from build123d import *

# Parameters (mm, degrees)
SKETCH_1_R          = 10
SKETCH_1_R_2        = 3.5
SKETCH_1_R_3        = 1.5
EXTRUDE_1_DEPTH     = 3
SKETCH_2_R          = 10
SKETCH_2_R_2        = 4.5
SKETCH_2_R_3        = 1.5
CUT_EXTRUDE_1_DEPTH = 1


with BuildPart() as part:
    # 草图1 → 凸台-拉伸1 (new body)
    with BuildSketch(Plane(origin=(0, 0, 0), x_dir=(1, 0, 0), z_dir=(0, 1, 0))):
        Circle(SKETCH_1_R)
        Circle(SKETCH_1_R_2, mode=Mode.SUBTRACT)
        with Locations((0, 6.5)):
            Circle(SKETCH_1_R_3, mode=Mode.SUBTRACT)
        with Locations((0, -6.5)):
            Circle(SKETCH_1_R_3, mode=Mode.SUBTRACT)
        with Locations((-6.5, 0)):
            Circle(SKETCH_1_R_3, mode=Mode.SUBTRACT)
        with Locations((6.5, 0)):
            Circle(SKETCH_1_R_3, mode=Mode.SUBTRACT)
    extrude(amount=EXTRUDE_1_DEPTH)

    # 草图2 → 切除-拉伸1 (cut)
    with BuildSketch(Plane(origin=(0, 3, 0), x_dir=(1, 0, 0), z_dir=(0, 1, 0))):
        Circle(SKETCH_2_R)
        Circle(SKETCH_2_R_2, mode=Mode.SUBTRACT)
        with Locations((0, -6.5)):
            Circle(SKETCH_2_R_3, mode=Mode.SUBTRACT)
        with Locations((0, 6.5)):
            Circle(SKETCH_2_R_3, mode=Mode.SUBTRACT)
        with Locations((6.5, 0)):
            Circle(SKETCH_2_R_3, mode=Mode.SUBTRACT)
        with Locations((-6.5, 0)):
            Circle(SKETCH_2_R_3, mode=Mode.SUBTRACT)
    extrude(amount=-CUT_EXTRUDE_1_DEPTH, mode=Mode.SUBTRACT)


solid = part.part
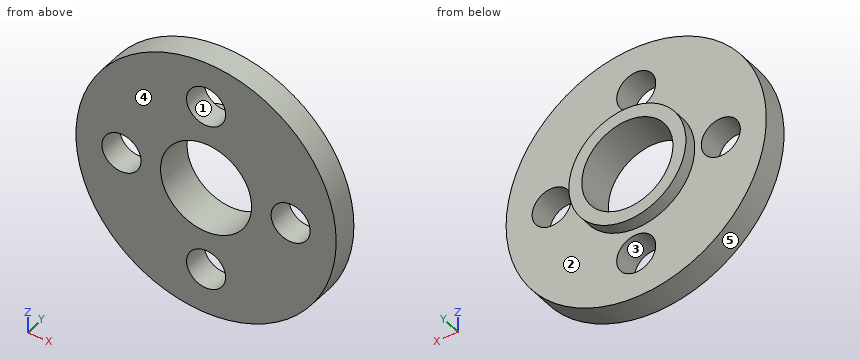
Design review of the part built by this model. Coordinates are the model's own, in mm. Face numbers are marked on the shaded views. A direction names the side the tool comes from. Coordinates: 2 decimals unless noted, no trailing zeros. Loops run counter-clockwise (first coordinate to the right, second up) from the corner with the lowest first, then second, coordinate; pieces in that order, holes last. Notation, with made-up numbers: (43, -36) -> (65, -36) arc R21 cw to (65, -29) -> close; hole circle Ø3 at (-29, -36). An arc over 180 degrees is marked (long way). Use a Markdown table: item, result. Add a question column.
Item 1: Clearance check with flat-ended pins moving along their axes: P1, Ø1.5, axis at x = 0.5, z = 6.5, coming from the +Y side; P2, Ø4, axis at x = 3, z = 7.5, coming from the +Y side; P3, Ø1, axis at y = 0.5, z = 4, coming from the +X side; P4, Ø1, axis at y = 0.5, z = -8, coming from the -X side. State where each tip first meets the part, or that it passes through.
Item 2: We need section B-B, the plane x = 0. Write out the cut boundary in (y, z).
Item 3: The part is to be moulded in two halves that separate along Z. For the marked faces 3, 4 and 5, say which applies: +Z half, -Z half, draft (parallel to the pull), parting line (faces both ways), or undercut.
Item 4: Wall thickness on L1, parallel to Z at x = 0, y = 1.85; L2, parallel to Z at x = 0, y = 2.05: over which ranges is each line inside the solid? List them lowest first. Write a range as from..to.
Item 5: We need section C-C, the plane y = 0.5. Write out the cut boundary in (x, z), and give its area (3 significant figures).
Item 6: We need section D-D, the plane z = -7.25. Write out the cut boundary in (x, y), and give its area (3 significant figures).
Item 7: We need section A-A, the plane z = 0. Write out the cut boundary in (x, y), and give its area (3 significant figures).
Item 8: Machinability: for the marked faces 1 and 2, which of the approach directions +Z, -Z, +X, -X, +Y, -Y give a long, thin tool a straight path to every point of the face, cutting with its end or side? Answer none if there is none.
Numbers:
| question | item | result |
|---|---|---|
| 1 | P1 | passes through |
| 1 | P2 | stops at y = 2 |
| 1 | P3 | stops at x = 9.37 |
| 1 | P4 | stops at x = -6.61 |
| 2 | outline | (0, -10) -> (2, -10) -> (2, -8) -> (0, -8) -> close; (0, -5) -> (2, -5) -> (2, -4.5) -> (3, -4.5) -> (3, -3.5) -> (0, -3.5) -> close; (0, 3.5) -> (3, 3.5) -> (3, 4.5) -> (2, 4.5) -> (2, 5) -> (0, 5) -> close; (0, 8) -> (2, 8) -> (2, 10) -> (0, 10) -> close |
| 3 | face 3 | undercut |
| 3 | face 4 | draft |
| 3 | face 5 | parting line |
| 4 | L1 | z = -10..-8, -5..-3.5, 3.5..5, 8..10 |
| 4 | L2 | z = -4.5..-3.5, 3.5..4.5 |
| 5 | outline | circle Ø20 at (0, 0); hole circle Ø3 at (-6.5, 0); hole circle Ø7 at (0, 0); hole circle Ø3 at (0, -6.5); hole circle Ø3 at (0, 6.5); hole circle Ø3 at (6.5, 0) |
| 5 | area | 247 mm^2 |
| 6 | outline | (-6.89, 0) -> (-1.3, 0) -> (-1.3, 2) -> (-6.89, 2) -> close; (1.3, 0) -> (6.89, 0) -> (6.89, 2) -> (1.3, 2) -> close |
| 6 | area | 22.4 mm^2 |
| 7 | outline | (-10, 0) -> (-8, 0) -> (-8, 2) -> (-10, 2) -> close; (-5, 0) -> (-3.5, 0) -> (-3.5, 3) -> (-4.5, 3) -> (-4.5, 2) -> (-5, 2) -> close; (3.5, 0) -> (5, 0) -> (5, 2) -> (4.5, 2) -> (4.5, 3) -> (3.5, 3) -> close; (8, 0) -> (10, 0) -> (10, 2) -> (8, 2) -> close |
| 7 | area | 16.0 mm^2 |
| 8 | face 1 | +Y, -Y |
| 8 | face 2 | +Y |
